The figure shows three views and two pictorial views of one solid part (mm, origin at its lowest corner). Answer the questions. A direction names the side the tool comes from. Give positions to 0.01 mm unless a question says otherwise; leave off trailing zeros. Write each loop counter-clockwise with the first axis right and the second up, starting at its lowest first coordinate (ties: lowest second). Pieces come first, ordered by that corner, then holes. Notation, with made-up numbers: (-10.75, -1) - (26.25, -1) arc R34 cw to (26.25, 32) - close; hole circle Ø2 at (47.5, 28.25). An arc over 180 degrees is marked (long way). Answer as CSV lines item,"result". Start each with the question number.
(1) For a pull along Y with two mould halves and no side action, classify the marked faces 1, 2, 3 and 4 as pulls with the +Y half, pulls with the -Y half, needs draft (parallel to the pull), parting line crosses it, or undercut.
(2) Find section C-C (z = 32). Write down the section's boundary in (x, y), then the cut area to 3 significant figures.
(3) Find section A-A (z = 16). Write down the section's boundary in (x, y).
(4) Find section D-D (y = 16). Write down the section's boundary in (x, z), then the cut area to 3 significant figures.
(5) Straight lines are drawn through the part: probe 1 along X at (y, z) = (27, 80.5); probe 2 along Y at (x, z) = (0.65, 16); probe 3 along Z at (x, y) = (0.7, 16). For each, find the intervals that lie inside material, in ascending order.
(6) Find section B-B (x = 19.5). Write down the section's boundary in (y, z), then the cut area to 3 significant figures.
(7) For the marked faces 5 and 6, determine the directions among +Z, -Z, +X, -X, +Y, -Y from which every point of the face is accessible in a straight line to the end or side of a thin tool.
(8) Each of these flat-tipped pins is pushed along its axis until it touches: pin 1 Ø12 at (x, y) = (18, 10.5) entering from +Z; pin 2 Ø1.5 at (y, z) = (28, 102.5) entering from -X. Where does it stop, or does it pass through?
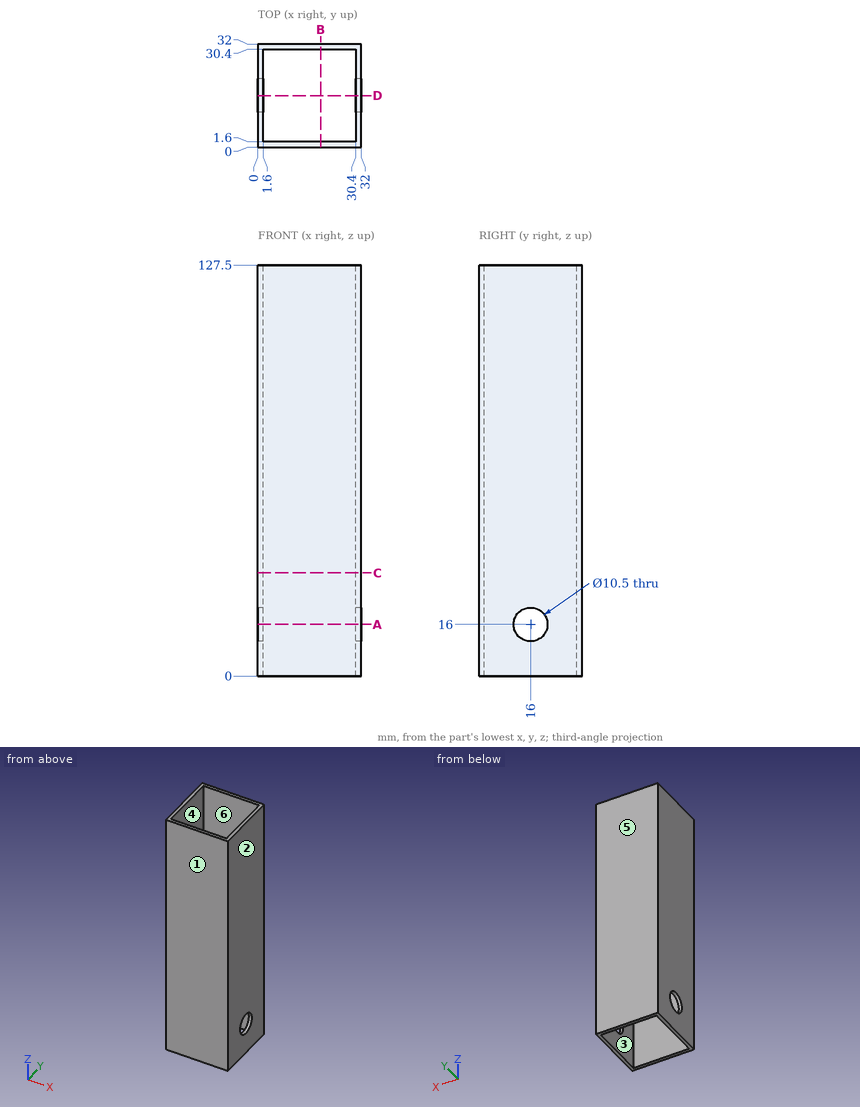
Result set:
1,face 1,"pulls with the -Y half"
1,face 2,"needs draft"
1,face 3,"undercut"
1,face 4,"undercut"
2,outline,"(0, 0) - (32, 0) - (32, 32) - (0, 32) - close; hole (1.6, 1.6) - (30.4, 1.6) - (30.4, 30.4) - (1.6, 30.4) - close"
2,area,"195 mm^2"
3,outline,"(0, 0) - (32, 0) - (32, 10.75) - (30.4, 10.75) - (30.4, 1.6) - (1.6, 1.6) - (1.6, 10.75) - (0, 10.75) - close; (0, 21.25) - (1.6, 21.25) - (1.6, 30.4) - (30.4, 30.4) - (30.4, 21.25) - (32, 21.25) - (32, 32) - (0, 32) - close"
4,outline,"(0, 0) - (1.6, 0) - (1.6, 10.75) - (0, 10.75) - close; (0, 21.25) - (1.6, 21.25) - (1.6, 127.5) - (0, 127.5) - close; (30.4, 0) - (32, 0) - (32, 10.75) - (30.4, 10.75) - close; (30.4, 21.25) - (32, 21.25) - (32, 127.5) - (30.4, 127.5) - close"
4,area,"374 mm^2"
5,probe 1,"0 to 1.6, 30.4 to 32"
5,probe 2,"0 to 10.75, 21.25 to 32"
5,probe 3,"0 to 10.75, 21.25 to 127.5"
6,outline,"(0, 0) - (1.6, 0) - (1.6, 127.5) - (0, 127.5) - close; (30.4, 0) - (32, 0) - (32, 127.5) - (30.4, 127.5) - close"
6,area,"408 mm^2"
7,face 5,"+Z, -Z, +X, -X, +Y"
7,face 6,"+Z, -Z"
8,pin 1,"through"
8,pin 2,"x = 0"
